The drawing under review shows one solid part. Ordinate dimensions are in mm from its lowest x, y, z. Coordinates: 2 decimals unless noted, no trailing zeros. Loops run counter-clockwise (first coordinate to the right, second up) from the corner with the lowest first, then second, coordinate; pieces in that order, holes last. Notation, with made-up numbers: M 68.5,88 L 81.5,88 A15 cw 81.5,107 Z; hole C 60,-28 d10. An arc over 180 degrees is marked long. Return JSON: item names as keys, results as strings.
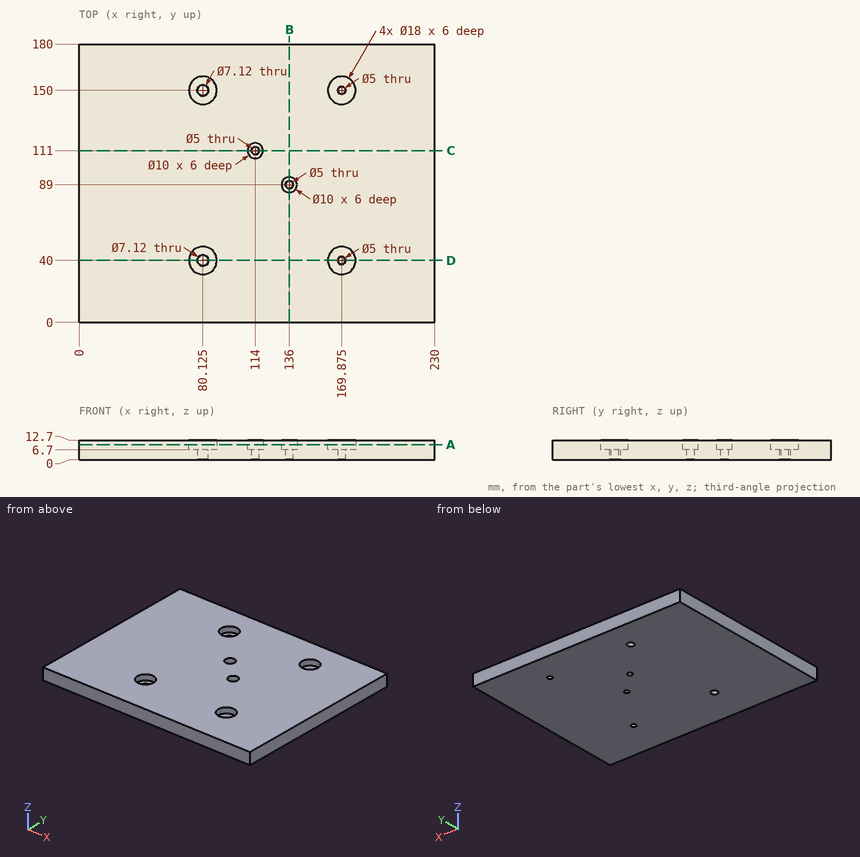
1. To check wall thickness, follow line 1 (Y direction, x = 136, z = 8.4); line 2 (X direction, y = 37.5, z = 7); line 3 (Y direction, x = 75.5, z = 9). State the ranges of each line that lie inside material, in increasing order.
Check values:
{"line 1": "0 to 84, 94 to 180", "line 2": "0 to 71.48, 88.77 to 161.23, 178.52 to 230", "line 3": "0 to 32.28, 47.72 to 142.28, 157.72 to 180"}
2. Add section D-D on y = 40. Give the boundary of the cut face in (x, z) (3 decimals).
Check values:
{"outline": "M 0,0 L 76.565,0 L 76.565,6.7 L 71.125,6.7 L 71.125,12.7 L 0,12.7 Z; M 83.685,0 L 167.375,0 L 167.375,6.7 L 160.875,6.7 L 160.875,12.7 L 89.125,12.7 L 89.125,6.7 L 83.685,6.7 Z; M 172.375,0 L 230,0 L 230,12.7 L 178.875,12.7 L 178.875,6.7 L 172.375,6.7 Z"}
3. Add section B-B on x = 136. Give the boundary of the cut face in (y, z), plus the area to 3 significant figures.
Check values:
{"outline": "M 0,0 L 86.5,0 L 86.5,6.7 L 84,6.7 L 84,12.7 L 0,12.7 Z; M 91.5,0 L 180,0 L 180,12.7 L 94,12.7 L 94,6.7 L 91.5,6.7 Z", "area": "2,190 mm²"}
4. Add section A-A on z = 10. Give the boundary of the cut face in (x, y) (3 decimals).
Check values:
{"outline": "M 0,0 L 230,0 L 230,180 L 0,180 Z; hole C 80.125,40 d18; hole C 80.125,150 d18; hole C 114,111 d10; hole C 136,89 d10; hole C 169.875,40 d18; hole C 169.875,150 d18"}
5. Add section C-C on y = 111. Give the boundary of the cut face in (x, z).
Check values:
{"outline": "M 0,0 L 111.5,0 L 111.5,6.7 L 109,6.7 L 109,12.7 L 0,12.7 Z; M 116.5,0 L 230,0 L 230,12.7 L 119,12.7 L 119,6.7 L 116.5,6.7 Z"}
6. Insertion check: pin 1 Ø9 at (x, y) = (168.5, 41.5) entering from +Z. The pin has a flat end and moves straight along its axis. Give the tip position at first contact, or say it passes through.
Check values:
{"pin 1": "z = 6.7"}
